Part print with two shaded views. Sizes in mm from the minimum x, y, z corner. A direction names the side the tool comes from. Coordinates: 2 decimals unless noted, no trailing zeros. Order: outer loops, then holes, each group sorted by start corner. A loop starts at its lowest first (then second) coordinate and runs counter-clockwise, first axis right, second up. Notation, with made-up numbers: (-25.75, -38.5) - (2.25, -38.5) arc R18 cw to (2.25, -24.5) - close; hole circle Ø4 at (33, -14). An arc over 180 degrees is marked (long way). Return JSON: item names as keys, results as strings.
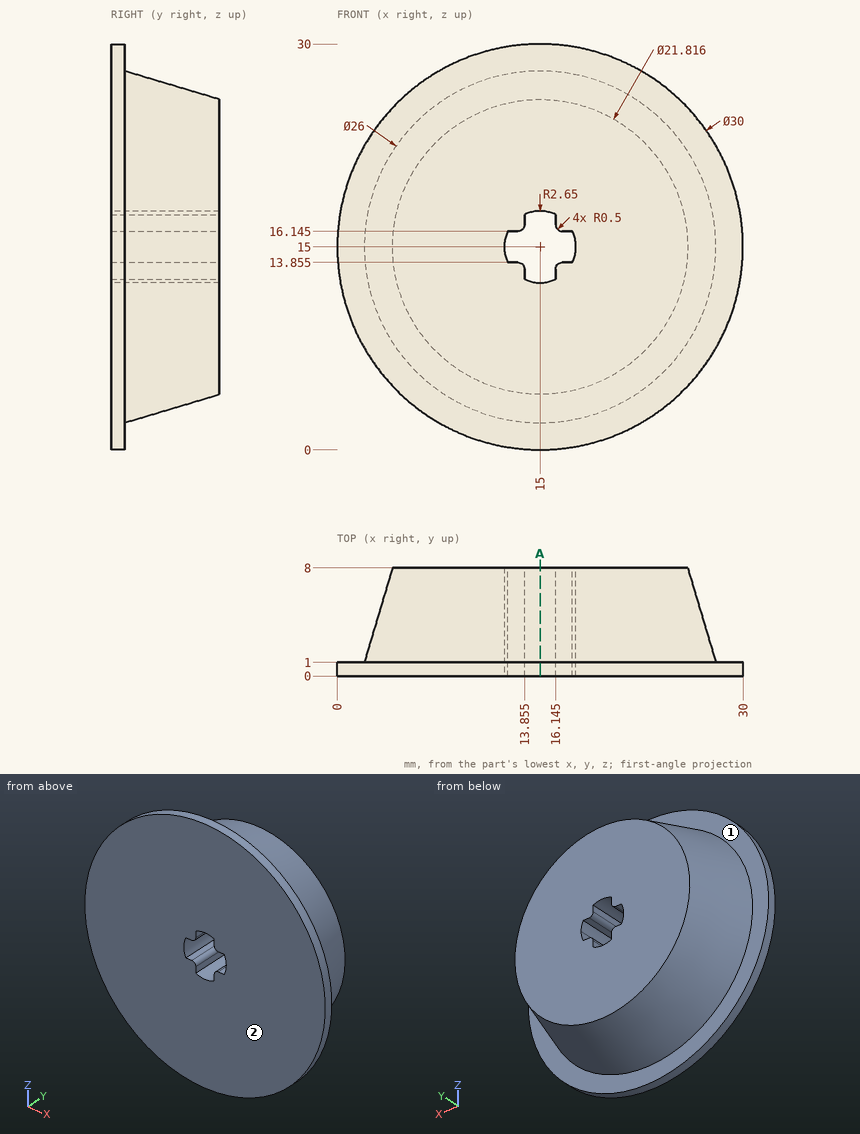
Item 1: Band-saw the part on A-A, the plane x = 15. List the corners of the cut face in (y, z).
Findings below:
{"outline": "(0, 0) - (1, 0) - (1, 2) - (8, 4.09) - (8, 12.35) - (0, 12.35) - close; (0, 17.65) - (8, 17.65) - (8, 25.91) - (1, 28) - (1, 30) - (0, 30) - close"}
Item 2: Which spindle directions (+Z, -Z, +X, -X, +Y, -Y) get a long thin tool onto all of the face, cutting with end or side? Do the marked faces 1 and 2. Say none if no direction does.
Findings below:
{"face 1": "+Y", "face 2": "+Z, -Z, +X, -X, -Y"}
Item 3: Wall check: L1, parallel to Y at x = 12.5, z = 2; L2, parallel to Z at x = 24.25, y = 6.25 (1 decimal); L3, parallel to X at y = 3.75, z = 5.5. Give the ranges that are in metal, low to high. Write a range as [from, to].
Findings below:
{"L1": "y = [0, 1]", "L2": "z = [8.3, 21.7]", "L3": "x = [7.38, 22.62]"}
Item 4: Drop flat-ended pins along their axis: P1, Ø0.6, axis at y = 2.5, z = 13, coming from the +X side; P2, Ø0.6, axis at y = 3.5, z = 13, coming from the -X side; P3, Ø0.6, axis at y = 5.5, z = 17, coming from the -X side; P4, Ø2, axis at x = 24, z = 10, coming from the -Y side. Give the stop position or say it passes through.
Findings below:
{"P1": "stops at x = 27.49", "P2": "stops at x = 2.81", "P3": "stops at x = 3.41", "P4": "stops at y = 0"}
